Autodesk Inventor part; units mm, degrees
ref_plane "YZ Plane" through (0, 0, 0) normal (1, 0, 0) x (0, 1, 0)
ref_plane "XZ Plane" through (0, 0, 0) normal (0, 1, 0) x (-1, 0, 0)
ref_plane "XY Plane" through (0, 0, 0) normal (0, 0, 1) x (1, 0, 0)
sketch "Sketch1" plane through (0, 0, 0) normal (1, 0, 0) x (0, 1, 0)
  line L0 (0, 0) -> (2.696, 0)
  line L1 (2.696, 0) -> (2.696, 6.6)
  circle A0 centre (2.696, 6.6) radius 0.5
  line L2 (-0.5, 0.5) -> (0.5, 0.5)
  line L3 (0.5, 0.5) -> (0.5, -0.5)
  line L4 (0.5, -0.5) -> (-0.5, -0.5)
  line L5 (-0.5, -0.5) -> (-0.5, 0.5)
  line L6 (-0.5, 0.5) -> (0.5, -0.5) construction
  line L7 (0.5, 0.5) -> (-0.5, -0.5) construction
  line L8 (0.5, -0.5) -> (3.1627, 6.4205)
  line L9 (-0.5, 0.5) -> (2.2374, 6.7993)
  dimension "d0" = 2.696
  dimension "d1" = 6.6
  dimension "d2" = 1
  dimension "d3" = 1
  dimension "d4" = 1
extrude "Extrusion1" add sketch "Sketch1" along normal blind 1 contours L3 L2 L9 A0 L1 L8 L0 | L3 L4 L5 L2 | L0 L8 L3 | L1 A0 L8 | A0
sketch "Sketch2" plane through (0, 0, 0) normal (-1, 0, 0) x (0, 0, 1)
  line L0 (-0.5, -0.5) -> (0.5, -0.5)
  line L1 (0.5, -0.5) -> (0.5, 0.5)
  line L2 (0.5, 0.5) -> (-0.5, 0.5)
  line L3 (-0.5, 0.5) -> (-0.5, -0.5)
  line L4 (-0.5, -0.5) -> (0.5, 0.5) construction
  line L5 (0.5, -0.5) -> (-0.5, 0.5) construction
  arc A0 (6.7993, 2.2374) -> (6.4205, 3.1627) centre (6.6, 2.696) ccw
  circle A1 centre (6.6, 2.696) radius 0.5
  point P0 (0, 0)
  point P1 (6.4205, 3.1627)
  point P2 (6.7993, 2.2374)
  dimension "d7" = 1
  dimension "d8" = 1
extrude "Extrusion2" add sketch "Sketch2" along normal blind 9.53
properties part number "Radius_Bone1_Joint"
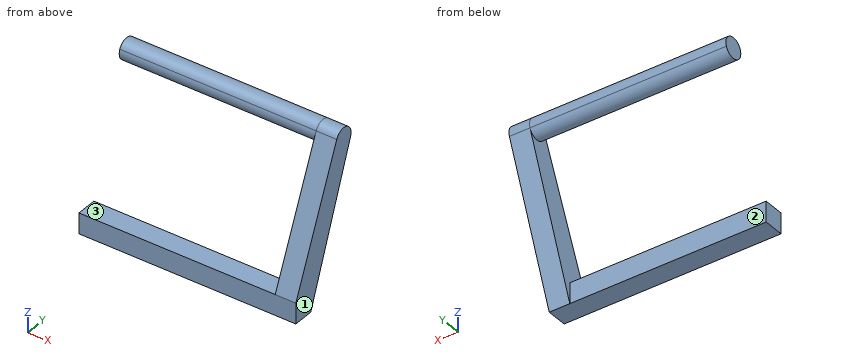
Model file for the job. Use its own axes, mm. Face numbers are marked on the shaded views. A direction names the side the tool comes from. Round coordinates to 2 decimals unless told otherwise and drop trailing zeros. Order: outer loops, then holes, each group sorted by start corner. A loop starts at its lowest first (then second) coordinate and runs counter-clockwise, first axis right, second up. Notation, with made-up numbers: M 35.25,30 L 88.25,30 A16 ccw 88.25,61 Z; hole C 58.25,-4 d3. An arc over 180 degrees is marked long. Write each question's results on one line, items separated by ' | '. Start each with the question number.
(1) Probe probe 1 along Y at (x, z) = (-6, 0.25); probe 2 along X at (y, z) = (2.35, 5.25). List the from-to ranges inside material, lowest first. Write a range as from..to.
(2) Drop a flat-ended pin along its axis: pin 1 (0.8 mm diameter, centred on x = -4, y = 0, fed in from +Z). Give the stop position or say it passes through.
(3) Saw through at A-A, the plane x = -6.5. Give the cut face in (y, z).
(4) Saw through at B-B, the plane z = 6.6. Give the cut face in (x, y).
(5) Saw through at C-C, the plane y = 2.05. Give the cut face in (x, z), then the cut area to 3 significant figures.
(6) Which spindle directions (+Z, -Z, +X, -X, +Y, -Y) get a long thin tool onto all of the face, cutting with end or side? Do the marked faces 1, 2 and 3. Say none if no direction does.
(7) Saw through at D-D, the plane x = 0.25. Give the cut face in (y, z).
Established:
1) probe 1: y = -0.5..0.5 | probe 2: x = 0..1
2) pin 1: stops at z = 0.5
3) outline: M -0.5,-0.5 L 0.5,-0.5 L 0.5,0.5 L -0.5,0.5 Z; M 2.24,6.8 A0.5 ccw long 3.16,6.42 A0.5 ccw Z
4) outline: M -9.53,2.2 L 0,2.2 L 0,2.15 L 1,2.15 L 1,3.2 L -9.53,3.2 Z
5) outline: M 0,3.53 L 1,3.53 L 1,6.37 L 0,6.37 Z | area: 2.84 mm^2
6) face 1: +Z, -Z, +X, +Y, -Y | face 2: +Z, -Z, -X, +Y | face 3: +Z, -X, +Y, -Y
7) outline: M -0.5,-0.5 L 0.5,-0.5 L 3.16,6.42 A0.5 ccw 2.24,6.8 L -0.5,0.5 Z
